from build123d import *

# Parameters (mm, degrees)
SKETCH1_W                = 95
SKETCH1_H                = 6
HOLE1_D                  = 120
F_9_16_CLEARANCE_HOLE1_D = 15
F_9_16_CLEARANCE_HOLE2_D = 15
CHAMFER1_SIZE            = 0.5
CHAMFER2_SIZE            = 1


with BuildPart() as part:
    # Sketch1 → Revolve1 (revolve)
    with BuildSketch(Plane.XY):
        with Locations((47.5, 2)):
            Rectangle(SKETCH1_W, SKETCH1_H)
    revolve(axis=Axis((0, 5, 0), (0, -1, 0)))

    # Hole1 (through all)
    with Locations(Plane(origin=(0, -1, 0), x_dir=(-1, 0, 0), z_dir=(0, -1, 0))):
        with Locations((0, 0)):
            Hole(HOLE1_D / 2)

    # 9/16 Clearance Hole1 (through all)
    with Locations(Plane(origin=(0, -1, 0), x_dir=(-1, 0, 0), z_dir=(0, -1, 0))):
        with Locations((69.282032303, 40), (0, 80)):
            Hole(F_9_16_CLEARANCE_HOLE1_D / 2)

    # 9/16 Clearance Hole2 (through all)
    with Locations(Plane(origin=(0, 5, 0), x_dir=(1, 0, 0), z_dir=(0, 1, 0))):
        with Locations((-69.282032303, -40), (69.282032303, 40), (69.282032303, -40), (0, -80)):
            Hole(F_9_16_CLEARANCE_HOLE2_D / 2)

    # Chamfer1
    chamfer1_edges = [part.edges().sort_by_distance(p)[0] for p in [
        (-7.5, -1, -80),
        (-7.5, 5, -80),
        (-76.782032303, -1, -40),
        (-76.782032303, 5, -40),
        (7.5, 5, 80),
        (7.5, -1, 80),
        (76.782032303, 5, 40),
        (76.782032303, -1, 40),
        (76.782032303, 5, -40),
        (76.782032303, -1, -40),
        (-61.782032303, 5, 40),
        (-61.782032303, -1, 40),
    ]]
    chamfer(chamfer1_edges, length=CHAMFER1_SIZE)

    # Chamfer2
    chamfer2_edges = [part.edges().sort_by_distance(p)[0] for p in [
        (-95, -1, 0),
        (-95, 5, 0),
    ]]
    chamfer(chamfer2_edges, length=CHAMFER2_SIZE)


solid = part.part
Geometry check sheet. Reference: the model listing, model coordinates, mm. Round coordinates to 2 decimals unless told otherwise and drop trailing zeros. Order: outer loops, then holes, each group sorted by start corner. A loop starts at its lowest first (then second) coordinate and runs counter-clockwise, first axis right, second up. Notation, with made-up numbers: M 71,-27 L 105,-27 A11 ccw 105,-15 Z; hole C -32,44.5 d5. An arc over 180 degrees is marked long. Answer in a Markdown table with one row per item.
(1) Go/stop test with flat-tipped pins: P1, Ø9, axis at x = 69.28, z = 40, coming from the -Y side; P2, Ø2, axis at y = 1.5, z = -40.5, coming from the -X side. Record where each tip stops, or that it passes through.
Responses:
| item | result |
|---|---|
| P1 | passes through |
| P2 | stops at x = -86.4 |
(2) Sectioned sample at B-B, the plane y = 0.9. Record the cut outline in (x, z), and give its area (3 significant figures).
Responses:
| item | result |
|---|---|
| outline | C 0,0 d190; hole C -69.28,-40 d15; hole C -69.28,40 d15; hole C 0,0 d120; hole C 0,-80 d15; hole C 0,80 d15; hole C 69.28,-40 d15; hole C 69.28,40 d15 |
| area | 16,000 mm² |
(3) Draft check along X on faces 1 (the face through (70.91, 1.96, 47.32)), 2 (the face through (-61, -1, 1)), 3 (the face through (-20.59, 2.03, -92.74)). Enter one of: released by +X, released by -X, zero draft, split by the parting line, or undercut.
Responses:
| item | result |
|---|---|
| face 1 | undercut |
| face 2 | zero draft |
| face 3 | split by the parting line |
(4) Scan lines: probe 1 along Z at (x, y) = (0, 2.25); probe 2 along Z at (x, y) = (-69.5, 2.5); probe 3 along Z at (x, y) = (-68, 0.75). Record each from-to range of solid material in increasing order. Write a range as from..to.
Responses:
| item | result |
|---|---|
| probe 1 | z = -95..-87.5, -72.5..-60, 60..72.5, 87.5..95 |
| probe 2 | z = -64.77..-47.5, -32.5..32.5, 47.5..64.77 |
| probe 3 | z = -66.34..-47.39, -32.61..32.61, 47.39..66.34 |
(5) Sectioned sample at A-A, the plane z = 0. Record the cut outline in (x, y).
Responses:
| item | result |
|---|---|
| outline | M -95,0 L -94,-1 L -60,-1 L -60,5 L -94,5 L -95,4 Z; M 60,-1 L 94,-1 L 95,0 L 95,4 L 94,5 L 60,5 Z |
(6) Sectioned sample at C-C, the plane z = 40. State how many separate pieces and enclosed holes the cut face has, and give its area (3 significant figures).
Responses:
| item | result |
|---|---|
| separate pieces | 4 |
| enclosed holes | 0 |
| area | 314 mm² |
